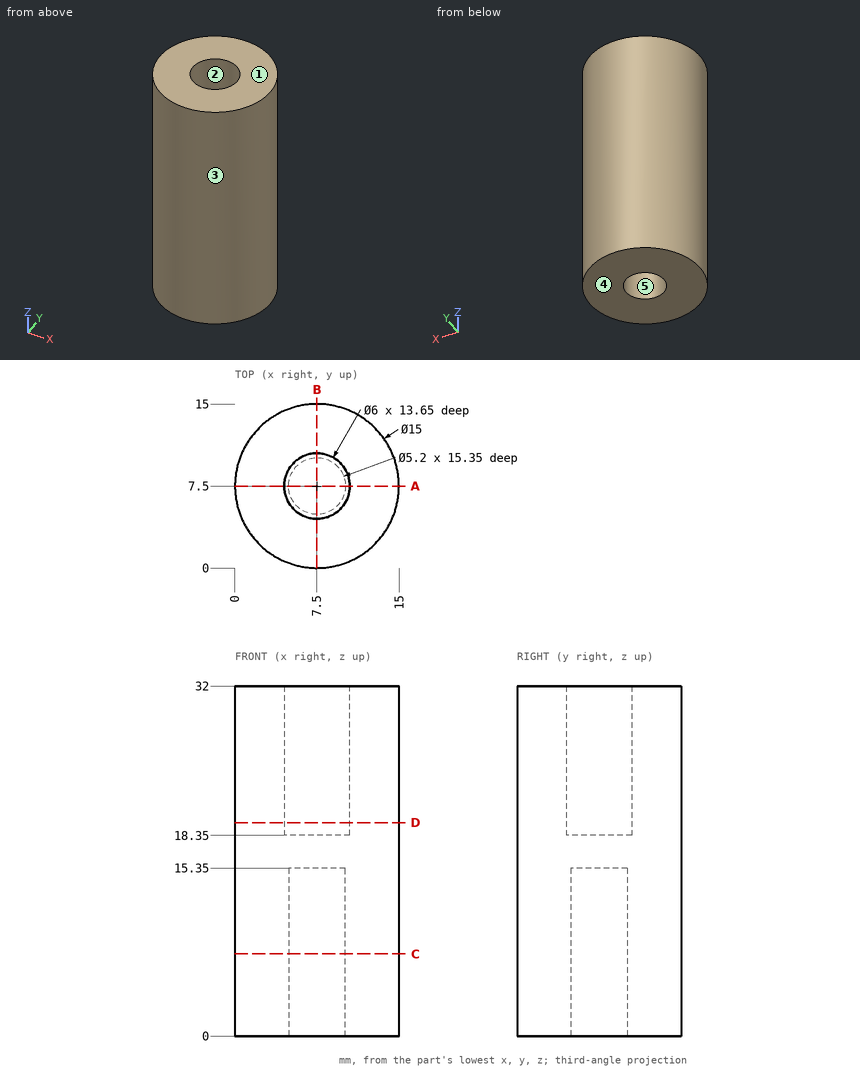
Input: dimensioned drawing with shaded views. Units: mm. Origin: part minimum x, y, z. A direction names the side the tool comes from. Give positions to 0.01 mm unless a question says otherwise; leave off trailing zeros. Write each loop counter-clockwise with the first axis right and the second up, starting at its lowest first coordinate (ties: lowest second). Pieces come first, ordered by that corner, then holes. Notation, with made-up numbers: (65.25, -31) -> (109.25, -31) arc R21 cw to (109.25, 2) -> close; hole circle Ø4 at (59, -17). An arc over 180 degrees is marked (long way). Answer as a JSON object with one key per item and string values.
1. Cut plane C-C on z = 7.5. Output: boundary loops of the cut face in (x, y).
Ans:
{"outline": "circle Ø15 at (7.5, 7.5); hole circle Ø5.2 at (7.5, 7.5)"}
2. Contact query for flat-ended pins moving along their axis: pin 1 (4.5 mm diameter, centred on x = 7.5, y = 7.5, fed in from -Z); pin 2 (1.5 mm diameter, centred on y = 2, z = 18, fed in from -X); pin 3 (4 mm diameter, centred on y = 11, z = 10.5, fed in from +X). Output: stop coordinate, or through.
Ans:
{"pin 1": "stops at z = 15.35", "pin 2": "stops at x = 1.7", "pin 3": "stops at x = 14.85"}
3. Cut plane A-A on y = 7.5. Output: boundary loops of the cut face in (x, z), and give its area (3 significant figures).
Ans:
{"outline": "(0, 0) -> (4.9, 0) -> (4.9, 15.35) -> (10.1, 15.35) -> (10.1, 0) -> (15, 0) -> (15, 32) -> (10.5, 32) -> (10.5, 18.35) -> (4.5, 18.35) -> (4.5, 32) -> (0, 32) -> close", "area": "318 mm^2"}
4. Cut plane D-D on z = 19.5. Output: boundary loops of the cut face in (x, y), and give its area (3 significant figures).
Ans:
{"outline": "circle Ø15 at (7.5, 7.5); hole circle Ø6 at (7.5, 7.5)", "area": "148 mm^2"}
5. Ray query, probe 1 along Y at (x, z) = (7.5, 5.25); probe 2 along X at (y, z) = (6, 4.5); probe 3 along Y at (x, z) = (7.5, 23.5). Return the intervals inside material, ascending. Write a range as from..to.
Ans:
{"probe 1": "y = 0..4.9, 10.1..15", "probe 2": "x = 0.15..5.38, 9.62..14.85", "probe 3": "y = 0..4.5, 10.5..15"}
6. Access query for the marked faces 1 and 2. Directions: +Z, -Z, +X, -X, +Y, -Y. A direction counts if a zero-diameter tool reaches every point of the face in a straight line with its end or side. Return the directions, or none.
Ans:
{"face 1": "+Z, +X, -X, +Y, -Y", "face 2": "+Z"}
7. Mould query, pull axis X, two halves, no side actions, for the marked faces 3, 4 and 5. Classes: pulls with the +X half, pulls with the -X half, needs draft (parallel to the pull), parting line crosses it, or undercut.
Ans:
{"face 3": "parting line crosses it", "face 4": "needs draft", "face 5": "undercut"}
